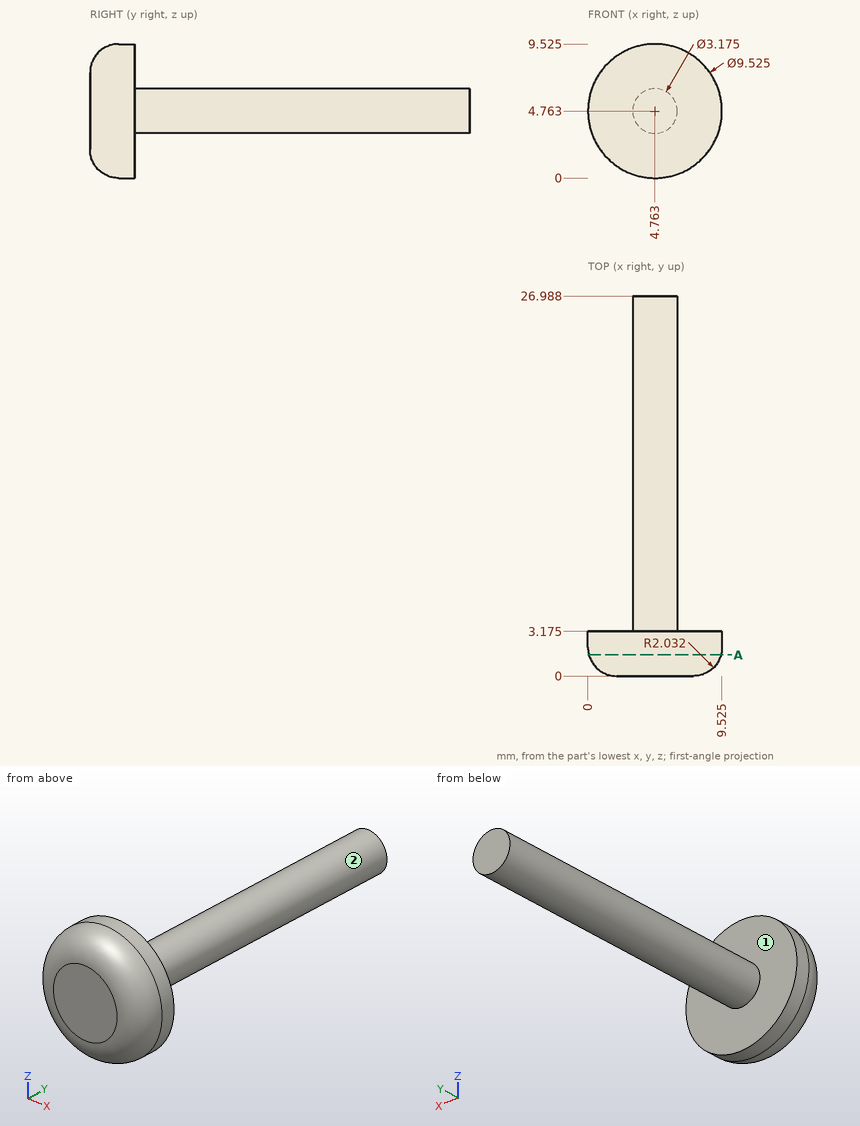
Source: three-view drawing plus pictorial views. Frame: mm from the lowest corner of the part. Coordinates: 2 decimals unless noted, no trailing zeros. Loops run counter-clockwise (first coordinate to the right, second up) from the corner with the lowest first, then second, coordinate; pieces in that order, holes last. Notation, with made-up numbers: (-11.75, 67.25) -> (21.25, 67.25) arc R29 cw to (21.25, 106.25) -> close; hole circle Ø4 at (66, -27.75). An arc over 180 degrees is marked (long way). Answer in a Markdown table with one row per item. Add a question column.
Q1. Ray query, line 1 along Y through (x, z) = (5, 6.75) (1 decimal); line 2 along Z through (x, y) = (5.5, 4.75) (1 decimal); line 3 along X through (y, z) = (21.5, 6) (1 decimal). Return the intervals inside material, ascending.
Q2. Contact query for flat-ended pins moving along their axis: pin 1 Ø4 at (y, z) = (24, 8) entering from +X (1 decimal); pin 2 Ø2 at (x, z) = (6.5, 2.5) entering from -Y; pin 3 Ø3 at (y, z) = (4.5, 6.5) entering from -X. Output: stop coordinate, or through.
Q3. Section A-A on y = 1.5. Return the cut outline in (x, z) (1 decimal).
Q4. Pull-direction query (X, two-part tool) for the marked faces 1 and 2; classes: pulls with the +X half, pulls with the -X half, needs draft (parallel to the pull), parting line crosses it, or undercut.
Computed values:
| question | item | result |
|---|---|---|
| 1 | line 1 | y = 0 to 3.2 |
| 1 | line 2 | z = 3.4 to 6.2 |
| 1 | line 3 | x = 3.8 to 5.8 |
| 2 | pin 1 | stops at x = 5.8 |
| 2 | pin 2 | stops at y = 0 |
| 2 | pin 3 | stops at x = 0.11 |
| 3 | outline | circle Ø9.4 at (4.8, 4.8) |
| 4 | face 1 | needs draft |
| 4 | face 2 | parting line crosses it |
